Geometry: final body of the model. Coordinates: model frame, mm. A direction names the side the tool comes from. Give positions to 0.01 mm unless a question says otherwise; leave off trailing zeros. Write each loop counter-clockwise with the first axis right and the second up, starting at its lowest first coordinate (ties: lowest second). Pieces come first, ordered by that corner, then holes. Notation, with made-up numbers: M 16.25,42 L 24.25,42 A21 ccw 24.25,47 Z; hole C 52.25,46.25 d9. An arc over 180 degrees is marked long. Use a Markdown table: item, result. Add a question column.
1) Draft query along Z for faces 1 (the cylindrical face through (36.25, 21.79, 4.23)), 2 (the cylindrical face through (-157.206, -19.855, -1.24)), 3 (the cylindrical face through (-27.83, -13.9, -1.71)), 4 (the flat face through (-222.273, -35, 6)). Return one class per face: +Z half, -Z half, draft (parallel to the pull), parting line (faces both ways), or undercut.
2) Line query: line 1 (Y direction, x = -143, z = 0); line 2 (Y direction, x = 17, z = 1.75); line 3 (Z direction, x = -85, y = -23.5). Output: solid intervals per line, ascending.
3) Section B-B on x = -102.5. Return the cut outline in (y, z) (3 decimals).
4) Pin query (flat end, axial travel): pin 1 (6 mm diameter, centred on x = -28, z = 4.5, fed in from -Y); pin 2 (1.5 mm diameter, centred on y = -29, z = 5.5, fed in from +X); pin 3 (3 mm diameter, centred on x = -11, y = -4.5, fed in from -Z). Return the tip coordinate at first contact, or that it passes through.
5) Set-up query: faces 5 (the cylindrical face through (-157.206, -21.492, -1.025)), 6 (the cylindrical face through (36.25, 5.85, -2.06)), 7 (the flat face through (45.216, 8, 4)). Return all of +Z, -Z, +X, -X, +Y, -Y with unobstructed straight access to the full face (end or side cutting, diameter ignored); none if empty.
6) Section A-A on z = 0. Return the cut outline in (x, y) (3 decimals).
```python
from build123d import *

# Parameters (mm, degrees)
SKETCH5_R   = 9.525
SKETCH5_R_2 = 7.874


with BuildPart() as part:
    # Sweep1: sweep along a path in Sketch4
    with BuildLine(Plane.XY) as sweep1_path:
        Line((45.216188471, 15.150806357), (27.533916935, 15.150806357))
        ThreePointArc((27.533916935, 15.150806357), (7.811905698, 12.55435432), (-10.566083065, 4.941942125))
        Line((-10.566083065, 4.941942125), (-52.191198388, -19.090329412))
        ThreePointArc((-52.191198388, -19.090329412), (-70.569187152, -26.702741607), (-90.291198388, -29.299193643))
        Line((-90.291198388, -29.299193643), (-222.273469925, -29.299193643))
    # Sketch5 → Sweep1 (sweep)
    with BuildSketch(Plane(origin=(45.216188471, 15.150806357, 0), x_dir=(0, 0, 1), z_dir=(-1, 0, 0))):
        Circle(SKETCH5_R)
        Circle(SKETCH5_R_2, mode=Mode.SUBTRACT)
    sweep(path=sweep1_path.line)


solid = part.part
```
Found:
| question | item | result |
|---|---|---|
| 1 | face 1 | undercut |
| 1 | face 2 | parting line |
| 1 | face 3 | undercut |
| 1 | face 4 | draft |
| 2 | line 1 | -38.82 to -37.17, -21.43 to -19.77 |
| 2 | line 2 | 4.95 to 6.66, 22.16 to 23.86 |
| 2 | line 3 | -7.7 to -5.53, 5.53 to 7.7 |
| 3 | outline | C -29.299,0 d19.05; hole C -29.299,0 d15.748 |
| 4 | pin 1 | y = -17.07 |
| 4 | pin 2 | x = -52.45 |
| 4 | pin 3 | z = -7 |
| 5 | face 5 | -X |
| 5 | face 6 | +X |
| 5 | face 7 | +Z, -Z, +X, +Y, -Y |
| 6 | outline | M -222.273,-38.824 L -90.291,-38.824 A85.725 ccw -47.429,-27.339 L -5.804,-3.307 A66.675 cw 27.534,5.626 L 45.216,5.626 L 45.216,7.277 L 27.534,7.277 A68.326 ccw -6.629,-1.877 L -48.254,-25.909 A84.074 cw -90.291,-37.173 L -222.273,-37.173 Z; M -222.273,-21.425 L -90.291,-21.425 A68.326 ccw -56.128,-12.271 L -14.503,11.761 A84.074 cw 27.534,23.025 L 45.216,23.025 L 45.216,24.676 L 27.534,24.676 A85.725 ccw -15.329,13.191 L -56.954,-10.841 A66.675 cw -90.291,-19.774 L -222.273,-19.774 Z |
